Autodesk Inventor part; units mm, degrees
ref_plane "YZ Plane" through (0, 0, 0) normal (1, 0, 0) x (0, 1, 0)
ref_plane "XZ Plane" through (0, 0, 0) normal (0, 1, 0) x (-1, 0, 0)
ref_plane "XY Plane" through (0, 0, 0) normal (0, 0, 1) x (1, 0, 0)
sketch "Sketch1" plane through (0, 0, 0) normal (0, 1, 0) x (-1, 0, 0)
  line L0 (-37, -97) -> (37, -97)
  line L1 (37, -97) -> (37, 97)
  line L2 (37, 97) -> (-37, 97)
  line L3 (-37, 97) -> (-37, -97)
  line L4 (-37, -97) -> (37, 97) construction
  line L5 (37, -97) -> (-37, 97) construction
  point P0 (0, 0)
  dimension "d0" = 74
  dimension "d1" = 194
extrude "Extrusion1" add sketch "Sketch1" against normal blind 3
sketch "Sketch2" plane through (0, -3, 0) normal (0, -1, 0) x (1, 0, 0)
  line L0 (-37, 97) -> (-37, -97)
  line L1 (-37, -97) -> (37, -97)
  line L2 (37, -97) -> (37, 97)
  line L3 (37, 97) -> (-37, 97)
  line L4 (34, 94) -> (-34, 94)
  line L5 (-34, 94) -> (-34, -94)
  line L6 (-34, -94) -> (34, -94)
  line L7 (34, -94) -> (34, 94)
  line L8 (34, 94) -> (-34, -94) construction
  line L9 (-34, 94) -> (34, -94) construction
  point P0 (0, 0)
  dimension "d4" = 3
  dimension "d5" = 3
extrude "Extrusion2" add sketch "Sketch2" along normal blind 3 contours L7 L6 L5 L4
fillet "Fillet1" radius 2 8 edges at (34, -4.5, 94) (-34, -4.5, 94) (37, -1.5, 97) (-37, -1.5, 97) (34, -4.5, -94) (37, -1.5, -97) (-34, -4.5, -94) (-37, -1.5, -97)
fillet "Fillet2" radius 0.5 8 edges at (-33.4142, -6, 93.4142) (-34, -6, 0) (-33.4142, -6, -93.4142) (0, -6, -94) (33.4142, -6, -93.4142) (34, -6, 0) (33.4142, -6, 93.4142) (0, -6, 94)
properties part number "module-lid_command"
The listing builds one solid part. Answer for the finished solid, in the listing's coordinates (mm). Round coordinates to 2 decimals unless told otherwise and drop trailing zeros. Order: outer loops, then holes, each group sorted by start corner. A loop starts at its lowest first (then second) coordinate and runs counter-clockwise, first axis right, second up. Notation, with made-up numbers: (29, 46) - (83, 46) arc R25 ccw to (83, 83) - close; hole circle Ø2 at (-9.75, 45.5). An arc over 180 degrees is marked (long way). Put each result on its own line as item: value. Start each with the question number.
(1) Find section C-C (z = 73). Give the vertices of the cut face in (x, y).
(2) Find section A-A (y = -4.5). Give the vertices of the cut face in (x, z).
(3) Given P1, Ø2, axis at x = 6, y = -4.5, coming from the +Z side; P2, Ø10, axis at x = -5, z = 30.5, coming from the +Y side; P3, Ø0.8, axis at x = 10, y = -3.5, coming from the -Z side; P4, Ø2, axis at y = -4.5, z = -10.5, coming from the +X side, each flat-ended and moving along its own axis, determine where each tip first touches the part or whether it passes through.
(4) Straight lines are drawn through the part: probe 1 along X at (y, z) = (-5, -43); probe 2 along Z at (x, y) = (-19.5, -5.5). For each, find the intervals that lie inside material, in ascending order. Write a range as from..to.
(5) Find section B-B (x = 18.5). Give the vertices of the cut face in (y, z), plus the area to 3 significant figures.
Reply:
1. outline: (-37, -3) - (-34, -3) - (-34, -5.5) arc R0.5 ccw to (-33.5, -6) - (33.5, -6) arc R0.5 ccw to (34, -5.5) - (34, -3) - (37, -3) - (37, 0) - (-37, 0) - close
2. outline: (-34, -92) arc R2 ccw to (-32, -94) - (32, -94) arc R2 ccw to (34, -92) - (34, 92) arc R2 ccw to (32, 94) - (-32, 94) arc R2 ccw to (-34, 92) - close
3. P1: z = 94
3. P2: y = 0
3. P3: z = -94
3. P4: x = 34
4. probe 1: -34..34
4. probe 2: -94..94
5. outline: (-6, -93.5) arc R0.5 ccw to (-5.5, -94) - (-3, -94) - (-3, -97) - (0, -97) - (0, 97) - (-3, 97) - (-3, 94) - (-5.5, 94) arc R0.5 ccw to (-6, 93.5) - close
5. area: 1,150 mm^2
